Geometry: final body of the model. Coordinates: model frame, mm. A direction names the side the tool comes from. Give positions to 0.01 mm unless a question says otherwise; leave off trailing zeros. Order: outer loops, then holes, each group sorted by start corner. A loop starts at its lowest first (then second) coordinate and runs counter-clockwise, first axis right, second up. Notation, with made-up numbers: (70, 8.5) - (125, 8.5) arc R24 cw to (125, 19.5) - close; hole circle Ø9 at (15, 76). An arc over 180 degrees is marked (long way). Put each result on its own line as item: value. Start each with the question number.
1. Ray query, line 1 along Y through (x, z) = (3, -0.5); line 2 along Y through (x, z) = (2.2, 0) (3 decimals); line 3 along X through (y, z) = (13, 0). Return the intervals inside material, ascending. Write a range as from..to.
2. Mould query, pull axis Y, two halves, no side actions, for faces 1 (the flat face through (-1, 2, -3)), 2 (the flat face through (1, 15.725, -1)), 3 (the flat face through (0, 0, -2)), 4 (the cylindrical face through (3.021, 9.304, -1.016)). Classes: pulls with the +Y half, pulls with the -Y half, needs draft (parallel to the pull), parting line crosses it, or undercut.
3. Set-up query: faces 5 (the flat face through (3.915, 0.986, 2.219)), 6 (the cylindrical face through (-1, 11, 0)), 7 (the cylindrical face through (3.91, 7.95, -0.92)), 8 (the cylindrical face through (0.45, -10.25, -1.43)), 9 (the flat face through (3.88, 0.99, -2.28)). Return all of +Z, -Z, +X, -X, +Y, -Y with unobstructed straight access to the full face (end or side cutting, diameter ignored); none if empty.
4. Section C-C on z = -2.5. Return the cut outline in (x, y) (3 decimals).
5. First-contact query: P1, Ø4, axis at x = -1, y = 8.5, coming from the +Z side; P2, Ø4, axis at x = 3, y = -16, coming from the +Z side; P3, Ø4, axis at y = -9.5, z = 1.5, coming from the +X side; P4, Ø6, axis at x = 1, y = 4, coming from the -Z side. Flat tips, straight axial feed; report the tip coordinate or a pass-through.
6. Section A-A on z = 0.5. Return the cut outline in (x, y) (1 decimal), plus the area to 3 significant figures.
7. Section B-B on y = -12.5. Return the cut outline in (x, z), plus the area to 3 significant figures.
8. Section D-D on z = -4. Return the cut outline in (x, y).
from build123d import *

# Parameters (mm, degrees)
SKETCH1_R                = 3
BOSS_EXTRUDE1_DEPTH      = 15.725
SKETCH2_R                = 1
CUT_EXTRUDE3_DEPTH       = 10.2
BOSS_EXTRUDE2_DEPTH      = 2
SKETCH4_R                = 1.5
BOSS_EXTRUDE3_DEPTH      = 20.8
BOSS_EXTRUDE4_DEPTH      = 2
BOSS_EXTRUDE4_DEPTH_BACK = 1
SKETCH6_R                = 2
SKETCH6_R_2              = 1.1
SKETCH7_R                = 1.1
CUT_EXTRUDE4_DEPTH       = 3


with BuildPart() as part:
    # Sketch1 → Boss-Extrude1 (new body)
    with BuildSketch(Plane(origin=(0, 0, 0), x_dir=(1, 0, 0), z_dir=(0, 1, 0))):
        with Locations(Location((0, 0, 0), (0, 0, 270))):
            Circle(SKETCH1_R)
    extrude(amount=BOSS_EXTRUDE1_DEPTH)

    # Sketch2 → Cut-Extrude3 (cut)
    with BuildSketch(Plane(origin=(0, 15.725, 0), x_dir=(1, 0, 0), z_dir=(0, 1, 0))):
        with Locations(Location((0, 0, 0), (0, 0, 270))):
            Circle(SKETCH2_R)
    extrude(amount=-CUT_EXTRUDE3_DEPTH, mode=Mode.SUBTRACT)

    # Sketch3 → Boss-Extrude2 (add)
    with BuildSketch(Plane(origin=(0, 0, 0), x_dir=(-1, 0, 0), z_dir=(0, -1, 0))):
        Polygon((5.196152423, 0), (2.598076211, 4.5), (-2.598076211, 4.5), (-5.196152423, 0), (-2.598076211, -4.5), (2.598076211, -4.5), align=None)
    extrude(amount=-BOSS_EXTRUDE2_DEPTH)

    # Sketch4 → Boss-Extrude3 (add)
    with BuildSketch(Plane(origin=(0, 0, 0), x_dir=(-1, 0, 0), z_dir=(0, -1, 0))):
        with Locations(Location((0, 0, 0), (0, 0, 90))):
            Circle(SKETCH4_R)
    extrude(amount=BOSS_EXTRUDE3_DEPTH)

    # Sketch6 → Boss-Extrude4 (add, two sides: drawn at the far end of the back side and taken through both)
    with BuildSketch(Plane(origin=(3, 0, 0), x_dir=(0, 0, -1), z_dir=(1, 0, 0)).offset(-BOSS_EXTRUDE4_DEPTH_BACK)):
        with Locations((0, 9.725)):
            Circle(SKETCH6_R)
        with Locations((0, 9.725)):
            Circle(SKETCH6_R_2, mode=Mode.SUBTRACT)
    extrude(amount=BOSS_EXTRUDE4_DEPTH + BOSS_EXTRUDE4_DEPTH_BACK)

    # Sketch7 → Cut-Extrude4 (cut)
    with BuildSketch(Plane(origin=(3, 0, 0), x_dir=(0, 0, -1), z_dir=(1, 0, 0))):
        with Locations((0, 9.725)):
            Circle(SKETCH7_R)
    extrude(amount=-CUT_EXTRUDE4_DEPTH, mode=Mode.SUBTRACT)


solid = part.part
Resolved:
1. line 1: 0..2, 7.79..8.75, 10.7..11.66
1. line 2: 0..8.625, 10.825..15.725
1. line 3: -3..-1, 1..3
2. face 1: undercut
2. face 2: pulls with the +Y half
2. face 3: pulls with the -Y half
2. face 4: undercut
3. face 5: +Z, +X, -Y
3. face 6: +Y
3. face 7: +X
3. face 8: -Y
3. face 9: -Z, +X, -Y
4. outline: (-3.753, 0) - (3.753, 0) - (3.753, 2) - (1.658, 2) - (1.658, 15.725) - (-1.658, 15.725) - (-1.658, 2) - (-3.753, 2) - close
5. P1: z = 3
5. P2: z = 1.12
5. P3: x = 1.5
5. P4: z = -4.5
6. outline: (-4.9, 0) - (-1.4, 0) - (-1.4, -20.8) - (1.4, -20.8) - (1.4, 0) - (4.9, 0) - (4.9, 2) - (3, 2) - (3, 7.8) - (5, 7.8) - (5, 8.7) - (0.9, 8.7) - (0.9, 5.5) - (-0.9, 5.5) - (-0.9, 15.7) - (-3, 15.7) - (-3, 2) - (-4.9, 2) - close; (0.9, 10.7) - (5, 10.7) - (5, 11.7) - (3, 11.7) - (3, 15.7) - (0.9, 15.7) - close
6. area: 142 mm^2
7. outline: circle Ø3 at (0, 0)
7. area: 7.07 mm^2
8. outline: (-2.89, 0) - (2.89, 0) - (2.89, 2) - (-2.89, 2) - close
